from build123d import *

# Parameters (mm, degrees)
SKETCH_W     = 97.89
SKETCH_H     = 6.5
PAD_DEPTH    = 10.35
SKETCH001_R  = 0.4
POCKET_DEPTH = 70
PAD001_DEPTH = 5


with BuildPart() as part:
    # Sketch → Pad (new body)
    with BuildSketch(Plane.XY):
        Rectangle(SKETCH_W, SKETCH_H)
    extrude(amount=PAD_DEPTH)

    # Sketch001 (on Face6 of Pad) → Pocket (cut)
    with BuildSketch(Plane.XY.offset(10.35)):
        with Locations((3.81, 0)):
            Circle(SKETCH001_R)
        with Locations((6.35, 0)):
            Circle(SKETCH001_R)
        with Locations((-16.51, 0)):
            Circle(SKETCH001_R)
        with Locations((-13.97, 0)):
            Circle(SKETCH001_R)
        with Locations((-34.29, 0)):
            Circle(SKETCH001_R)
        with Locations((-36.83, 0)):
            Circle(SKETCH001_R)
        with Locations((13.97, 0)):
            Circle(SKETCH001_R)
        with Locations((16.51, 0)):
            Circle(SKETCH001_R)
        with Locations((24.13, 0)):
            Circle(SKETCH001_R)
        with Locations((26.67, 0)):
            Circle(SKETCH001_R)
        with Locations((34.29, 0)):
            Circle(SKETCH001_R)
        with Locations((36.83, 0)):
            Circle(SKETCH001_R)
        with Locations((44.45, 0)):
            Circle(SKETCH001_R)
        with Locations((46.99, 0)):
            Circle(SKETCH001_R)
        with Locations((-46.99, 0)):
            Circle(SKETCH001_R)
        with Locations((-44.45, 0)):
            Circle(SKETCH001_R)
        with Locations((-26.67, 0)):
            Circle(SKETCH001_R)
        with Locations((-24.13, 0)):
            Circle(SKETCH001_R)
        with Locations((-6.35, 0)):
            Circle(SKETCH001_R)
        with Locations((-3.81, 0)):
            Circle(SKETCH001_R)
    extrude(amount=-POCKET_DEPTH, mode=Mode.SUBTRACT)

    # Sketch002 (on Face4 of Pocket) → Pad001 (join)
    with BuildSketch(Plane(origin=(0, 0, 0), x_dir=(1, 0, 0), z_dir=(0, 0, -1))):
        with BuildLine():
            Line((-39.61, 2.2225), (-39.61, -2.22))
            ThreePointArc((-41.51, -2.22), (-40.56, -3.318203), (-39.61, -2.22))
            Line((-41.51, -2.22), (-41.51, 2.22))
            ThreePointArc((-39.61, 2.2225), (-40.561445, 3.319446), (-41.51, 2.22))
        make_face()
        with BuildLine():
            Line((41.51, 2.22), (41.51, -2.22))
            ThreePointArc((39.61, -2.22), (40.56, -3.318203), (41.51, -2.22))
            Line((39.61, -2.22), (39.61, 2.22))
            ThreePointArc((41.51, 2.22), (40.56, 3.318203), (39.61, 2.22))
        make_face()
    extrude(amount=PAD001_DEPTH)


solid = part.part
Model file for the job. Use its own axes, mm. Coordinates: 2 decimals unless noted, no trailing zeros. Write each loop counter-clockwise with the first axis right and the second up, starting at its lowest first coordinate (ties: lowest second). Pieces come first, ordered by that corner, then holes. Notation, with made-up numbers: (34, -18.5) - (77, -18.5) arc R28 ccw to (77, 1.5) - close; hole circle Ø7 at (42, 37). An arc over 180 degrees is marked (long way). Write each question's results on one line, items separated by ' | '. Start each with the question number.
1) Cut at B-B (z = 2.5). Count the separate pieces of the cut face and the enclosed holes in it, then the cut area to 3 significant figures.
2) Probe line 1 along X through (y, z) = (-1, -3); line 2 along Y through (x, z) = (6.35, 8); line 3 along Z through (x, y) = (-12.5, 1.5). List the from-to ranges inside material, lowest first. Write a range as from..to.
3) Flat gauge pins, fed straight in: P1, Ø2, axis at x = -7, z = 0.5, coming from the +Y side; P2, Ø3, axis at x = 1.5, y = -0.5, coming from the -Z side; P3, Ø2, axis at y = -0.5, z = -2, coming from the -X side; P4, Ø3, axis at x = -34, y = 0, coming from the +Z side. Where does each tip first touch, or does it go through?
4) Cut at C-C (x = 43). Write the cut outline in (y, z), then the cut area to 3 significant figures.
5) Mould opens along X. For faces 1 (the face through (-41, 0, -5)), 2 (the face through (-48.945, 0, 5)), 3 (the face through (-1, 0, 0)), 4 (the face through (-40.583, 3.318, -2.465)) say: pulls with the +X half, pulls with the -X half, needs draft (parallel to the pull), parting line crosses it, or undercut.
6) Cut at A-A (z = -1.25). Write the cut outline in (x, y).
Returned:
1) separate pieces: 1 | enclosed holes: 20 | area: 626 mm^2
2) line 1: -41.51..-39.61, 39.61..41.51 | line 2: -3.25..-0.4, 0.4..3.25 | line 3: 0..10.35
3) P1: y = 3.25 | P2: z = 0 | P3: x = -41.51 | P4: z = 10.35
4) outline: (-3.25, 0) - (3.25, 0) - (3.25, 10.35) - (-3.25, 10.35) - close | area: 67.3 mm^2
5) face 1: needs draft | face 2: pulls with the -X half | face 3: undercut | face 4: undercut
6) outline: (-41.51, -2.22) arc R0.96 ccw (long way) to (-39.61, -2.22) - (-39.61, 2.22) arc R0.96 ccw (long way) to (-41.51, 2.22) - close; (39.61, -2.22) arc R0.96 ccw (long way) to (41.51, -2.22) - (41.51, 2.22) arc R0.96 ccw (long way) to (39.61, 2.22) - close
